```python
from build123d import *

# Parameters (mm, degrees)
BOSS_EXTRUDE1_DEPTH = 3
SKETCH2_W           = 3
SKETCH2_H           = 11.487699198
CUT_EXTRUDE1_DEPTH  = 16


# Read off the part's stored shape, not the designer's step: Boss-Extrude1
with BuildPart() as part:
    # Boss-Extrude1 outline → Boss-Extrude1 (new body)
    with BuildSketch(Plane.XY):
        with BuildLine():
            Line((-95.687613819, 113.066263652), (-95.687613819, 103.066263652))
            Line((-95.687613819, 103.066263652), (-107.013116357, 103.066263652))
            add(Edge.make_bspline(
                [(-107.013116357, 103.066263652), (0, -103.066263652), (107.013116357, 103.066263652)],
                knots=[0.057157488, 0.057157488, 0.057157488, 0.942842512, 0.942842512, 0.942842512], degree=2))
            Line((107.013116357, 103.066263652), (95.68761382, 103.066263652))
            Line((95.68761382, 103.066263652), (95.68761382, 113.066263652))
            Line((95.68761382, 113.066263652), (84.362111282, 113.066263652))
            Line((84.362111282, 113.066263652), (84.362111282, 103.066263652))
            add(Edge.make_bspline(
                [(84.362111282, 103.066263652), (77.169203523, 89.870321464), (60.617973136, 63.983872026), (42.369102372, 42.101536817), (28.30806557, 30.298322138), (17.949926074, 24.101443082), (8.601675425, 20.762226356), (-2.4893e-05, 19.742494759), (-8.601757959, 20.762212203), (-17.949851697, 24.101471728), (-28.308921959, 30.298047433), (-39.552364136, 39.742329541), (-51.44403726, 52.605304358), (-63.778998477, 68.925840315), (-77.169000129, 89.870127882), (-84.362111282, 103.066263652)],
                knots=[0.078216729, 0.078216729, 0.078216729, 0.140190459, 0.22322343, 0.306256401, 0.361611715, 0.416967029, 0.472322343, 0.527677657, 0.583032971, 0.638388285, 0.693743599, 0.749098913, 0.804454227, 0.859809541, 0.921783758, 0.921783758, 0.921783758], degree=2))
            Line((-84.362111282, 103.066263652), (-84.362111282, 113.066263652))
            Line((-84.362111282, 113.066263652), (-95.687613819, 113.066263652))
        make_face()
    extrude(amount=BOSS_EXTRUDE1_DEPTH)

    # Sketch2 → Cut-Extrude1 (cut)
    with BuildSketch(Plane.XY):
        with Locations((0, 4.256150401)):
            Rectangle(SKETCH2_W, SKETCH2_H)
    extrude(amount=CUT_EXTRUDE1_DEPTH, mode=Mode.SUBTRACT)


solid = part.part
```
The model under review builds one solid part; all positions refer to its coordinate system, in mm. Round coordinates to 2 decimals unless told otherwise and drop trailing zeros. Order: outer loops, then holes, each group sorted by start corner. A loop starts at its lowest first (then second) coordinate and runs counter-clockwise, first axis right, second up. Notation, with made-up numbers: (-3.75, 66.25) -> (30.25, 66.25) arc R14 cw to (30.25, 90.25) -> close; hole circle Ø8 at (-21, -11). An arc over 180 degrees is marked (long way). One line per item, written item: value. Start each with the question number.
Q1. Wall thickness on line 1 (X direction, y = 77.5, z = 2.1); line 2 (X direction, y = 72.5, z = 2); line 3 (Y direction, x = -0.5, z = 1.5): over which ranges is each line inside the solid? List them lowest first.
Q2. Clearance check with flat-ended pins moving along their axes: pin 1 Ø0.9 at (y, z) = (107, 1.5) entering from +X; pin 2 Ø0.9 at (x, z) = (0, 1.5) entering from -Y. State where each tip first meets the part, or that it passes through.
Q3. Take a section at A-A (y = 106). Write out the cut boundary in (x, z).
Reported:
1. line 1: x = -92.8 to -69.26, 69.26 to 92.8
1. line 2: x = -89.75 to -65.96, 65.96 to 89.75
1. line 3: y = 10 to 20
2. pin 1: stops at x = 95.69
2. pin 2: stops at y = 10
3. outline: (-95.69, 0) -> (-84.36, 0) -> (-84.36, 3) -> (-95.69, 3) -> close; (84.36, 0) -> (95.69, 0) -> (95.69, 3) -> (84.36, 3) -> close
